```python
from build123d import *

# Parameters (mm, degrees)
BOSS_EXTRUDE1_DEPTH      = 3.18
BOSS_EXTRUDE1_DEPTH_BACK = 3.18
SKETCH1_W                = 1.64
SKETCH1_H                = 6.36
SKETCH2_R                = 2.5
BOSS_EXTRUDE2_DEPTH      = 2.79
SKETCH3_R                = 3.135
BOSS_EXTRUDE3_DEPTH      = 5
SKETCH4_W                = 1
SKETCH4_H                = 1
BOSS_EXTRUDE4_DEPTH      = 3.9
SKETCH5_R                = 0.68
BOSS_EXTRUDE5_DEPTH      = 3.9
SKETCH6_R                = 2.245
CUT_EXTRUDE1_DEPTH       = 2


with BuildPart() as part:
    # Sketch1 → Boss-Extrude1 (new, two sides: drawn at the far end of the back side and taken through both)
    with BuildSketch(Plane.XY.offset(-BOSS_EXTRUDE1_DEPTH_BACK)):
        Rectangle(SKETCH1_W, SKETCH1_H)
    extrude(amount=BOSS_EXTRUDE1_DEPTH + BOSS_EXTRUDE1_DEPTH_BACK)

    # Sketch2 → Boss-Extrude2 (add)
    with BuildSketch(Plane.ZY.offset(0.82)):
        Circle(SKETCH2_R)
    extrude(amount=BOSS_EXTRUDE2_DEPTH)

    # Sketch3 → Boss-Extrude3 (add)
    with BuildSketch(Plane.ZY.offset(3.61)):
        Circle(SKETCH3_R)
    extrude(amount=BOSS_EXTRUDE3_DEPTH)

    # Sketch4 → Boss-Extrude4 (add)
    with BuildSketch(Plane(origin=(0.82, 0, 0), x_dir=(0, 0, -1), z_dir=(1, 0, 0))):
        with Locations((-2.68, 2.68)):
            Rectangle(SKETCH4_W, SKETCH4_H)
        with Locations((2.68, 2.68)):
            Rectangle(SKETCH4_W, SKETCH4_H)
        with Locations((-2.68, -2.68)):
            Rectangle(SKETCH4_W, SKETCH4_H)
        with Locations((2.68, -2.68)):
            Rectangle(SKETCH4_W, SKETCH4_H)
    extrude(amount=BOSS_EXTRUDE4_DEPTH)

    # Sketch5 → Boss-Extrude5 (add)
    with BuildSketch(Plane(origin=(0.82, 0, 0), x_dir=(0, 0, -1), z_dir=(1, 0, 0))):
        Circle(SKETCH5_R)
    extrude(amount=BOSS_EXTRUDE5_DEPTH)

    # Sketch6 → Cut-Extrude1 (cut)
    with BuildSketch(Plane.ZY.offset(8.61)):
        Circle(SKETCH6_R)
    extrude(amount=-CUT_EXTRUDE1_DEPTH, mode=Mode.SUBTRACT)


solid = part.part
```
Build history of the part. All positions in model axes, mm. A direction names the side the tool comes from. Coordinates: 2 decimals unless noted, no trailing zeros. Write each loop counter-clockwise with the first axis right and the second up, starting at its lowest first coordinate (ties: lowest second). Pieces come first, ordered by that corner, then holes.
1. 3-axis set-ups, long thin cutter, end or side, ignore diameter. For faces 4 (the flat face through (3, 2.18, 3)), 5 (the cylindrical face through (-2.2, -2.44, -0.54)), 6 (the flat face through (3, -3, 2.18)), 7 (the cylindrical face through (2.74, 0.2, -0.65)): which of +Z, -Z, +X, -X, +Y, -Y reach the whole face in a straight line?
Answer block:
face 4: +Z, -Z, +X
face 5: none
face 6: +X, +Y, -Y
face 7: +X
2. Drop flat-ended pins along their axis: pin 1 (3 mm diameter, centred on y = -1.5, z = -1, fed in from +X); pin 2 (3 mm diameter, centred on x = -6, z = -0.5, fed in from +Y) (3 decimals); pin 3 (3 mm diameter, centred on x = -3, y = 2.5, fed in from +Z); pin 4 (1.9 mm diameter, centred on y = 0.5, z = -1, fed in from -X). Give the stop position or say it passes through.
Answer block:
pin 1: stops at x = 4.72
pin 2: stops at y = 3.135
pin 3: stops at z = 2.92
pin 4: stops at x = -6.61
3. Band-saw the part on C-C, the plane z = 0. Give the cut face in (x, y) (3 decimals), and give its area (3 significant figures).
Answer block:
outline: (-8.61, -3.135) - (-3.61, -3.135) - (-3.61, -2.5) - (-0.82, -2.5) - (-0.82, -3.18) - (0.82, -3.18) - (0.82, -0.68) - (4.72, -0.68) - (4.72, 0.68) - (0.82, 0.68) - (0.82, 3.18) - (-0.82, 3.18) - (-0.82, 2.5) - (-3.61, 2.5) - (-3.61, 3.135) - (-8.61, 3.135) - (-8.61, 2.245) - (-6.61, 2.245) - (-6.61, -2.245) - (-8.61, -2.245) - close
area: 52.1 mm2
4. Pull direction X, two halves, no side cores. Call faces 1 (the flat face through (3, 3, 2.18)), 2 (the flat face through (-0.82, -2.2, -1.5)), 3 (the flat face through (-6.61, 0, 0)): released by +X, released by -X, zero draft, split by the parting line, or undercut.
Answer block:
face 1: zero draft
face 2: undercut
face 3: released by -X
5. Band-saw the part on A-A, the plane x = 2.75. Give the cut face in (y, z).
Answer block:
outline: (-3.18, -3.18) - (-2.18, -3.18) - (-2.18, -2.18) - (-3.18, -2.18) - close; (-3.18, 2.18) - (-2.18, 2.18) - (-2.18, 3.18) - (-3.18, 3.18) - close; circle Ø1.36 at (0, 0); (2.18, -3.18) - (3.18, -3.18) - (3.18, -2.18) - (2.18, -2.18) - close; (2.18, 2.18) - (3.18, 2.18) - (3.18, 3.18) - (2.18, 3.18) - close
6. Drill centre lines: probe 1 along Y at (x, z) = (-7.5, 0) (3 decimals); probe 2 along Y at (x, z) = (4, -2.5); probe 3 along X at (y, z) = (-2, -2). Where is each one in solid material? Low to high.
Answer block:
probe 1: y = -3.135 to -2.245, 2.245 to 3.135
probe 2: y = -3.18 to -2.18, 2.18 to 3.18
probe 3: x = -8.61 to -3.61, -0.82 to 0.82
7. Band-saw the part on B-B, the plane y = 2.75. Give the cut face in (x, z), and give its area (3 significant figures).
Answer block:
outline: (-8.61, -1.51) - (-3.61, -1.51) - (-3.61, 1.51) - (-8.61, 1.51) - close; (-0.82, -3.18) - (4.72, -3.18) - (4.72, -2.18) - (0.82, -2.18) - (0.82, 2.18) - (4.72, 2.18) - (4.72, 3.18) - (-0.82, 3.18) - close
area: 33.3 mm2
